Verification items for the finished model (mm, model axes). Face numbers are marked on the shaded views. A direction names the side the tool comes from. Round coordinates to 2 decimals unless told otherwise and drop trailing zeros. Loops run counter-clockwise (first coordinate to the right, second up) from the corner with the lowest first, then second, coordinate; pieces in that order, holes last. Notation, with made-up numbers: M 49.25,39.25 L 72.25,39.25 A25 ccw 72.25,72.25 Z; hole C 60.5,69 d1. An arc over 180 degrees is marked long. Answer as CSV lines item,"result".
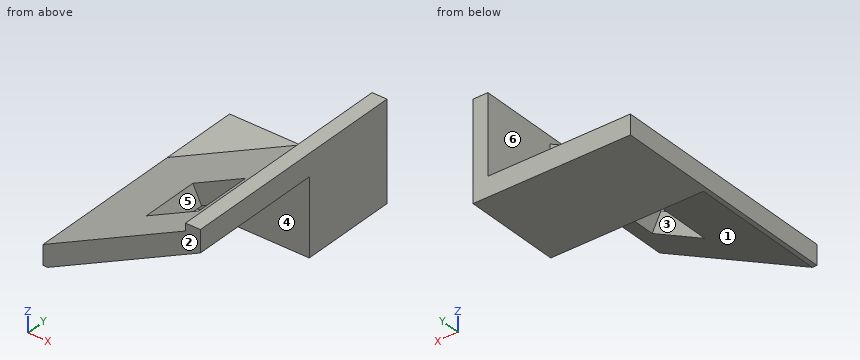
```python
from build123d import *

# Parameters (mm, degrees)
SKETCH1_W           = 50.8
SKETCH1_H           = 76.2
BOSS_EXTRUDE1_DEPTH = 6.35
SKETCH2_W           = 50.8
SKETCH2_H           = 50.8
BOSS_EXTRUDE2_DEPTH = 25.4
CUT_EXTRUDE1_REACH  = 52.8
SKETCH4_W           = 4.813703211
SKETCH4_H           = 76.2
BOSS_EXTRUDE3_DEPTH = 31.75
CUT_EXTRUDE2_DEPTH  = 44.45
CUT_EXTRUDE3_REACH  = 30.398
SKETCH6_W           = 19.05
SKETCH6_H           = 19.05


with BuildPart() as part:
    # Sketch1 → Boss-Extrude1 (new body)
    with BuildSketch(Plane.XY):
        with Locations((25.4, -38.1)):
            Rectangle(SKETCH1_W, SKETCH1_H)
    extrude(amount=BOSS_EXTRUDE1_DEPTH)

    # Sketch2 → Boss-Extrude2 (add)
    with BuildSketch(Plane.XY.offset(6.35)):
        with Locations((25.4, -50.8)):
            Rectangle(SKETCH2_W, SKETCH2_H)
    extrude(amount=BOSS_EXTRUDE2_DEPTH)

    # Sketch3 → Cut-Extrude1 (cut, up to next)
    with BuildSketch(Plane(origin=(0, -25.4, 0), x_dir=(1, 0, 0), z_dir=(0, 1, 0)), mode=Mode.PRIVATE) as cut_extrude1_sk1:
        Polygon((0, -6.35), (0, -31.75), (50.8, -31.75), align=None)
    cut_extrude1_tool1 = extrude(cut_extrude1_sk1.sketch, amount=-CUT_EXTRUDE1_REACH, mode=Mode.PRIVATE) & part.part
    add(cut_extrude1_tool1.solids().sort_by_distance((16.933333, -25.4, 23.283333))[0], mode=Mode.SUBTRACT)

    # Sketch4 → Boss-Extrude3 (add)
    with BuildSketch(Plane(origin=(0, 0, 0), x_dir=(-1, 0, 0), z_dir=(0, 0, -1))):
        with Locations((-48.393148395, -38.1)):
            Rectangle(SKETCH4_W, SKETCH4_H)
    extrude(amount=-BOSS_EXTRUDE3_DEPTH)

    # Sketch5 → Cut-Extrude2 (cut)
    with BuildSketch(Plane.XZ.offset(76.2)):
        Polygon((50.8, 0), (50.8, 24.650484171), (1.499031657, 0), align=None)
    extrude(amount=-CUT_EXTRUDE2_DEPTH, mode=Mode.SUBTRACT)

    # Sketch6 → Cut-Extrude3 (cut, up to next)
    with BuildSketch(Plane(origin=(-2.54, 0, 5.08), x_dir=(0.894427191, 0, 0.447213595), z_dir=(-0.447213595, 0, 0.894427191)), mode=Mode.PRIVATE) as cut_extrude3_sk1:
        with Locations((38.379049159, -53.975)):
            Rectangle(SKETCH6_W, SKETCH6_H)
    cut_extrude3_tool1 = extrude(cut_extrude3_sk1.sketch, amount=-CUT_EXTRUDE3_REACH, mode=Mode.PRIVATE) & part.part
    add(cut_extrude3_tool1.solids().sort_by_distance((31.787265, -53.975, 22.243633))[0], mode=Mode.SUBTRACT)


solid = part.part
```
1) Section check B-B (z = 14). Record the cut outline in (x, y), plus the area to 3 significant figures.
Here are the results:
outline,"M 15.3,-76.2 L 29.5,-76.2 L 29.5,-63.5 L 25.26,-63.5 L 25.26,-44.45 L 29.5,-44.45 L 29.5,-31.75 L 50.8,-31.75 L 50.8,0 L 45.99,0 L 45.99,-25.4 L 15.3,-25.4 Z"
area,"898 mm^2"
2) Section check A-A (y = -58). Record the cut outline in (x, z).
Here are the results:
outline,"M 0,0 L 1.5,0 L 26.11,12.3 L 23.27,17.98 L 0,6.35 Z; M 40.31,26.5 L 43.15,20.82 L 50.8,24.65 L 50.8,31.75 L 45.99,31.75 L 45.99,29.34 Z"
3) Draft check along Y on the marked faces 1, 2 and 3. Enter one of: +Y half, -Y half, draft (parallel to the pull), parting line (faces both ways), or undercut.
Here are the results:
face 1,"draft"
face 2,"-Y half"
face 3,"undercut"
4) Material ranges on probe 1 along Y at (x, z) = (32, 20.5); probe 2 along X at (y, z) = (-46, 30); probe 3 along Y at (x, z) = (39, 10.5), recorded low to high.
Here are the results:
probe 1,"y = -76.2 to -63.5, -44.45 to -25.4"
probe 2,"x = 45.99 to 50.8"
probe 3,"y = -31.75 to -25.4"
5) Section check D-D (x = 27). Record the cut outline in (y, z).
Here are the results:
outline,"M -76.2,12.75 L -63.5,12.75 L -63.5,19.85 L -76.2,19.85 Z; M -44.45,12.75 L -31.75,12.75 L -31.75,0 L 0,0 L 0,6.35 L -25.4,6.35 L -25.4,19.85 L -44.45,19.85 Z"
6) Go/stop test with flat-tipped pins: pin 1 (3 mm diameter, centred on y = -53, z = 17, fed in from +X); pin 2 (3 mm diameter, centred on y = -67, z = 19, fed in from +X); pin 3 (6 mm diameter, centred on x = 28, z = 5.5, fed in from -Y). Record where each tip stops, or that it passes through.
Here are the results:
pin 1,"stops at x = 24.51"
pin 2,"stops at x = 42.5"
pin 3,"stops at y = -31.75"
7) Set-up check for the marked faces 4, 5 and 6: record each of +Z, -Z, +X, -X, +Y, -Y from which the full face is reachable in a straight line by a thin tool's end or side.
Here are the results:
face 4,"-Z, +X, -Y"
face 5,"+Z, +X"
face 6,"+Z, -X, +Y"
8) Section check C-C (y = -28). Record the cut outline in (x, z), plus the area to 3 significant figures.
Here are the results:
outline,"M 0,0 L 50.8,0 L 50.8,31.75 L 45.99,31.75 L 45.99,29.34 L 0,6.35 Z"
area,"974 mm^2"
